from build123d import *

# Parameters (mm, degrees)
SKETCH2_W                                       = 115.292618629
SKETCH2_H                                       = 134.000000002
BOSS_EXTRUDE2_DEPTH                             = 8
FILLET2_R                                       = 6
CSK_FOR_M2_FLAT_HEAD_MACHINE_SCREW2_D           = 2.4
CSK_FOR_M2_FLAT_HEAD_MACHINE_SCREW2_CSINK_D     = 4.4
CSK_FOR_M2_FLAT_HEAD_MACHINE_SCREW2_CSINK_ANGLE = 90
CSK_FOR_M3_FLAT_HEAD_MACHINE_SCREW1_D           = 3.4
CSK_FOR_M3_FLAT_HEAD_MACHINE_SCREW1_CSINK_D     = 6.3
CSK_FOR_M3_FLAT_HEAD_MACHINE_SCREW1_CSINK_ANGLE = 90
SKETCH19_W                                      = 8
SKETCH19_H                                      = 99
BOSS_EXTRUDE3_DEPTH                             = 115.292618629
SKETCH21_W                                      = 135.292618629
SKETCH21_H                                      = 129
SKETCH21_W_2                                    = 115.292618629
SKETCH21_H_2                                    = 99
BOSS_EXTRUDE4_DEPTH                             = 8
FILLET3_R                                       = 5
CUT_EXTRUDE1_DEPTH                              = 4
SKETCH24_W                                      = 115.292618629
SKETCH24_H                                      = 10
BOSS_EXTRUDE5_DEPTH                             = 104
FILLET4_R                                       = 6
M2_5_CLEARANCE_HOLE1_D                          = 2.9
CUT_EXTRUDE4_START                              = -8
CUT_EXTRUDE4_DEPTH                              = 8
CHAMFER1_SIZE                                   = 0.9
SKETCH61_W                                      = 104
SKETCH61_H                                      = 10
CUT_EXTRUDE6_DEPTH                              = 115.292618629
SKETCH62_W                                      = 8
SKETCH62_H                                      = 129
CUT_EXTRUDE7_DEPTH                              = 135.292618629
F_5_6_5_6_DIAMETER_HOLE1_D                      = 5.6
F_5_6_5_6_DIAMETER_HOLE1_DEPTH                  = 8
F_5_6_5_6_DIAMETER_HOLE1_TIP                    = 1.682409733
SKETCH66_W                                      = 61.79
SKETCH66_H                                      = 30.000000002
CUT_EXTRUDE9_DEPTH                              = 8
SKETCH67_W                                      = 16.522618629
SKETCH67_H                                      = 30.000000002
CUT_EXTRUDE10_DEPTH                             = 8
FILLET5_R                                       = 6
FILLET6_R                                       = 3


with BuildPart() as part:
    # Sketch2 → Boss-Extrude2 (new body)
    with BuildSketch(Plane(origin=(0, 0, 0), x_dir=(1, 0, 0), z_dir=(0, 1, 0))):
        with Locations((4.853690686, 42.889279439)):
            Rectangle(SKETCH2_W, SKETCH2_H)
    extrude(amount=BOSS_EXTRUDE2_DEPTH)

    # Fillet2
    fillet2_edges = [part.edges().sort_by_distance(p)[0] for p in [
        (-52.792618629, 4, -109.88927944),
        (62.5, 4, -109.88927944),
    ]]
    fillet(fillet2_edges, radius=FILLET2_R)

    # CSK for M2 Flat Head Machine Screw2 (through all)
    with Locations(Plane(origin=(0, 0, 0), x_dir=(-1, 0, 0), z_dir=(0, -1, 0))):
        with Locations((-22.207381371, 75.889279438), (35.792618629, 75.889279438), (35.792618629, -10.110720562), (-22.207381371, -10.110720562)):
            CounterSinkHole(CSK_FOR_M2_FLAT_HEAD_MACHINE_SCREW2_D / 2, CSK_FOR_M2_FLAT_HEAD_MACHINE_SCREW2_CSINK_D / 2, counter_sink_angle=CSK_FOR_M2_FLAT_HEAD_MACHINE_SCREW2_CSINK_ANGLE)

    # CSK for M3 Flat Head Machine Screw1 (through all)
    with Locations(Plane(origin=(0, 8, 0), x_dir=(1, 0, 0), z_dir=(0, 1, 0))):
        with Locations((-48.662618629, 63.809279438), (8.227381371, 63.809279438), (8.227381371, -12.950720562), (-48.662618629, -12.950720562)):
            CounterSinkHole(CSK_FOR_M3_FLAT_HEAD_MACHINE_SCREW1_D / 2, CSK_FOR_M3_FLAT_HEAD_MACHINE_SCREW1_CSINK_D / 2, counter_sink_angle=CSK_FOR_M3_FLAT_HEAD_MACHINE_SCREW1_CSINK_ANGLE)

    # Sketch19 → Boss-Extrude3 (add)
    with BuildSketch(Plane.ZY.offset(52.792618629)):
        with Locations((28.110720562, 13.5)):
            Rectangle(SKETCH19_W, SKETCH19_H)
    extrude(amount=-BOSS_EXTRUDE3_DEPTH)

    # Sketch21 → Boss-Extrude4 (add)
    with BuildSketch(Plane.XY.offset(32.110720562)):
        with Locations((4.853690685, 8.5)):
            Rectangle(SKETCH21_W, SKETCH21_H)
        with Locations((4.853690686, 13.5)):
            Rectangle(SKETCH21_W_2, SKETCH21_H_2, mode=Mode.SUBTRACT)
    extrude(amount=-BOSS_EXTRUDE4_DEPTH)

    # Fillet3
    fillet3_edges = [part.edges().sort_by_distance(p)[0] for p in [
        (72.5, 73, 28.110720562),
        (72.5, -56, 28.110720562),
        (-62.792618629, -56, 28.110720562),
        (-62.792618629, 73, 28.110720562),
    ]]
    fillet(fillet3_edges, radius=FILLET3_R)

    # Sketch22 → Cut-Extrude1 (cut)
    with BuildSketch(Plane(origin=(0, 0, 24.110720562), x_dir=(-1, 0, 0), z_dir=(0, 0, -1))):
        with BuildLine():
            Line((62.792618629, -51), (62.792618629, 68))
            ThreePointArc((62.792618629, 68), (61.328152535, 71.535533906), (57.792618629, 73))
            Line((57.792618629, 73), (-67.5, 73))
            ThreePointArc((-67.5, 73), (-71.035533906, 71.535533906), (-72.5, 68))
            Line((-72.5, 68), (-72.5, -51))
            ThreePointArc((-72.5, -51), (-71.035533906, -54.535533906), (-67.5, -56))
            Line((-67.5, -56), (57.792618629, -56))
            ThreePointArc((57.792618629, -56), (61.328152535, -54.535533906), (62.792618629, -51))
        make_face()
        with BuildLine():
            Line((57.792618629, 69.75), (-67.5, 69.75))
            ThreePointArc((-67.5, 69.75), (-68.737436867, 69.237436867), (-69.25, 68))
            Line((-69.25, 68), (-69.25, -51))
            ThreePointArc((-69.25, -51), (-68.737436867, -52.237436867), (-67.5, -52.75))
            Line((-67.5, -52.75), (57.792618629, -52.75))
            ThreePointArc((57.792618629, -52.75), (59.030055496, -52.237436867), (59.542618629, -51))
            Line((59.542618629, -51), (59.542618629, 68))
            ThreePointArc((59.542618629, 68), (59.030055496, 69.237436867), (57.792618629, 69.75))
        make_face(mode=Mode.SUBTRACT)
    extrude(amount=-CUT_EXTRUDE1_DEPTH, mode=Mode.SUBTRACT)

    # Sketch24 → Boss-Extrude5 (add)
    with BuildSketch(Plane(origin=(0, 0, 24.110720562), x_dir=(-1, 0, 0), z_dir=(0, 0, -1))):
        with Locations((-4.853690686, 60)):
            Rectangle(SKETCH24_W, SKETCH24_H)
    extrude(amount=BOSS_EXTRUDE5_DEPTH)

    # Fillet4
    fillet4_edges = [part.edges().sort_by_distance(p)[0] for p in [
        (62.5, 60, -79.889279438),
        (-52.792618629, 60, -79.889279438),
    ]]
    fillet(fillet4_edges, radius=FILLET4_R)

    # M2.5 Clearance Hole1 (through all)
    with Locations(Plane(origin=(0, 8, 0), x_dir=(1, 0, 0), z_dir=(0, 1, 0))):
        with Locations((-28.27, 101.64), (-7.29, 101.64), (-7.29, 88.14), (-28.27, 88.14)):
            Hole(M2_5_CLEARANCE_HOLE1_D / 2)

    # Sketch60 → Cut-Extrude4 (cut)
    with BuildSketch(Plane(origin=(0, 8, 0), x_dir=(1, 0, 0), z_dir=(0, 1, 0)).offset(CUT_EXTRUDE4_START)):
        with BuildLine():
            Line((-30.27, 103.09), (-26.27, 103.09))
            ThreePointArc((-26.27, 103.09), (-24.82, 101.64), (-26.27, 100.19))
            Line((-26.27, 100.19), (-30.27, 100.19))
            ThreePointArc((-30.27, 100.19), (-31.72, 101.64), (-30.27, 103.09))
        make_face()
        with BuildLine():
            Line((-9.29, 103.09), (-5.29, 103.09))
            ThreePointArc((-5.29, 103.09), (-3.84, 101.64), (-5.29, 100.19))
            Line((-5.29, 100.19), (-9.29, 100.19))
            ThreePointArc((-9.29, 100.19), (-10.74, 101.64), (-9.29, 103.09))
        make_face()
        with BuildLine():
            Line((-30.27, 89.59), (-26.27, 89.59))
            ThreePointArc((-26.27, 89.59), (-24.82, 88.14), (-26.27, 86.69))
            Line((-26.27, 86.69), (-30.27, 86.69))
            ThreePointArc((-30.27, 86.69), (-31.72, 88.14), (-30.27, 89.59))
        make_face()
        with BuildLine():
            Line((-9.29, 89.59), (-5.29, 89.59))
            ThreePointArc((-5.29, 89.59), (-3.84, 88.14), (-5.29, 86.69))
            Line((-5.29, 86.69), (-9.29, 86.69))
            ThreePointArc((-9.29, 86.69), (-10.74, 88.14), (-9.29, 89.59))
        make_face()
    extrude(amount=CUT_EXTRUDE4_DEPTH, mode=Mode.SUBTRACT)

    # Chamfer1
    chamfer1_edges = [part.edges().sort_by_distance(p)[0] for p in [
        (-7.29, 8, -100.19),
        (-3.84, 8, -101.64),
        (-7.29, 8, -103.09),
        (-28.27, 8, -86.69),
        (-24.82, 8, -88.14),
        (-28.27, 8, -89.59),
        (-7.29, 8, -86.69),
        (-3.84, 8, -88.14),
        (-7.29, 8, -89.59),
        (-28.27, 8, -103.09),
        (-31.72, 8, -101.64),
        (-28.27, 8, -100.19),
        (-24.82, 8, -101.64),
        (-10.74, 8, -88.14),
        (-31.72, 8, -88.14),
        (-10.74, 8, -101.64),
    ]]
    chamfer(chamfer1_edges, length=CHAMFER1_SIZE)

    # Sketch61 → Cut-Extrude6 (cut)
    with BuildSketch(Plane.ZY.offset(52.792618629)):
        with Locations((-27.889279438, 60)):
            Rectangle(SKETCH61_W, SKETCH61_H)
    extrude(amount=-CUT_EXTRUDE6_DEPTH, mode=Mode.SUBTRACT)

    # Sketch62 → Cut-Extrude7 (cut)
    with BuildSketch(Plane.ZY.offset(62.792618629)):
        with Locations((28.110720562, 8.5)):
            Rectangle(SKETCH62_W, SKETCH62_H)
    extrude(amount=-CUT_EXTRUDE7_DEPTH, mode=Mode.SUBTRACT)

    # Ø5.6 (5.6) Diameter Hole1
    with Locations(Plane.XY.offset(24.110720562)):
        with Locations((-42.792618629, 4), (52.5, 4)):
            Hole(F_5_6_5_6_DIAMETER_HOLE1_D / 2, depth=F_5_6_5_6_DIAMETER_HOLE1_DEPTH)
            with Locations((0, 0, -(F_5_6_5_6_DIAMETER_HOLE1_DEPTH + F_5_6_5_6_DIAMETER_HOLE1_TIP / 2))):  # 118° drill point
                Cone(0, F_5_6_5_6_DIAMETER_HOLE1_D / 2, F_5_6_5_6_DIAMETER_HOLE1_TIP, mode=Mode.SUBTRACT)

    # Sketch66 → Cut-Extrude9 (cut)
    with BuildSketch(Plane.XZ):
        with Locations((31.605, -94.889279439)):
            Rectangle(SKETCH66_W, SKETCH66_H)
    extrude(amount=-CUT_EXTRUDE9_DEPTH, mode=Mode.SUBTRACT)

    # Sketch67 → Cut-Extrude10 (cut)
    with BuildSketch(Plane(origin=(0, 0, 0), x_dir=(-1, 0, 0), z_dir=(0, -1, 0))):
        with Locations((44.531309315, 94.889279439)):
            Rectangle(SKETCH67_W, SKETCH67_H)
    extrude(amount=-CUT_EXTRUDE10_DEPTH, mode=Mode.SUBTRACT)

    # Fillet5
    fillet5_edges = [part.edges().sort_by_distance(p)[0] for p in [
        (62.5, 4, -79.889279438),
        (0.71, 4, -109.88927944),
        (-36.27, 4, -109.88927944),
        (-52.792618629, 4, -79.889279438),
    ]]
    fillet(fillet5_edges, radius=FILLET5_R)

    # Fillet6
    fillet6_edges = [part.edges().sort_by_distance(p)[0] for p in [
        (0.71, 4, -79.889279438),
        (-36.27, 4, -79.889279438),
    ]]
    fillet(fillet6_edges, radius=FILLET6_R)


solid = part.part
Input: part model. Units: mm. Frame: model coordinates. A direction names the side the tool comes from. Round coordinates to 2 decimals unless told otherwise and drop trailing zeros. Loops run counter-clockwise (first coordinate to the right, second up) from the corner with the lowest first, then second, coordinate; pieces in that order, holes last. Notation, with made-up numbers: (10, -31.75) -> (58, -31.75) arc R19 cw to (58, -12.75) -> close; hole circle Ø1 at (72.5, -9). An arc over 180 degrees is marked (long way). Answer as a JSON object with one key per item and string values. Group by question number.
1) Section query B-B on x = 36. Output: boundary loops of the cut face in (y, z), plus the area to 3 significant figures.
2) Pin query (flat end, axial travel): pin 1 (3 mm diameter, centred on x = 17, z = -3.5, fed in from -Y); pin 2 (4 mm diameter, centred on y = 4.5, z = -96.5, fed in from +X); pin 3 (2.5 mm diameter, centred on y = 4, z = -88, fed in from -X). Return the tip coordinate at first contact, or that it passes through.
3) Draft query along X for faces 5 (the cylindrical face through (-37.172, 4.056, -80.745)), 6 (the flat face through (0.71, 4, -94)), 7 (the cylindrical face through (-31.72, 3.5, -101.61)). Return one class per face: +X half, -X half, draft (parallel to the pull), parting line (faces both ways), or undercut.
4) Reachability of faces 1 (the flat face through (30, 4, -79.889)), 2 (the cylindrical face through (-3.84, 3.5, -101.67)), 3 (the flat face through (-43, 4, -79.889)), 4 (the cylindrical face through (51.208, 1.516, 20.055)) from +Z, -Z, +X, -X, +Y, -Y: full face, straight path, thin tool, end or side. Return the list, or none.
5) Ray query, L1, parallel to X at y = 4, z = 20.75; L2, parallel to Z at x = -7.5, y = 7; L3, parallel to X at y = 2, z = -62.5. Return the intervals inside material, ascending.
6) Section query A-A on z = -101.64. Output: boundary loops of the cut face in (x, y).
Reply:
{
 "1": {"outline": "(0, -79.89) -> (8, -79.89) -> (8, 24.11) -> (0, 24.11) -> close", "area": "832 mm2"},
 "2": {"pin 1": "stops at y = 0", "pin 2": "stops at x = 0.71", "pin 3": "stops at x = -36.27"},
 "3": {"face 5": "-X half", "face 6": "+X half", "face 7": "undercut"},
 "4": {"face 1": "-Z, +X, +Y, -Y", "face 2": "+Y, -Y", "face 3": "-Z, -X, +Y, -Y", "face 4": "+Z"},
 "5": {"L1": "x = -52.79 to -45.59, -39.99 to 49.7, 55.3 to 62.5", "L2": "z = -109.89 to -103.09, -100.19 to -89.59, -86.69 to 24.11", "L3": "x = -52.79 to -49.75, -47.58 to 7.14, 9.31 to 62.5"},
 "6": {"outline": "(-36.27, 0) -> (-31.72, 0) -> (-31.72, 7.1) -> (-32.62, 8) -> (-36.27, 8) -> close; (-24.82, 0) -> (-10.74, 0) -> (-10.74, 7.1) -> (-11.64, 8) -> (-23.92, 8) -> (-24.82, 7.1) -> close; (-3.84, 0) -> (0.71, 0) -> (0.71, 8) -> (-2.94, 8) -> (-3.84, 7.1) -> close"}
}
